Input: part model. Units: mm. Frame: model coordinates. A direction names the side the tool comes from. Round coordinates to 2 decimals unless told otherwise and drop trailing zeros. Loops run counter-clockwise (first coordinate to the right, second up) from the corner with the lowest first, then second, coordinate; pieces in that order, holes last. Notation, with made-up numbers: (59, -9.75) - (108, -9.75) arc R8 ccw to (108, -1.75) - close; hole circle Ø4 at (68, 2). An arc over 180 degrees is marked (long way). One line per question, with ' | ' between items. Start each with the question number.
Item 1: Section B-B, the plane z = 17.25. Return loops of the section in (x, y).
Item 2: Set-up query: faces 5 (the face through (17.5, -2, 14)), 6 (the face through (20.05, 11.9, 0.49)), 7 (the face through (0, -5, 23)), 8 (the face through (10, -3.4, 1)), 9 (the face through (0, -3, 3)). Return all of +Z, -Z, +X, -X, +Y, -Y with unobstructed straight access to the full face (end or side cutting, diameter ignored); none if empty.
Item 3: Section C-C, the plane z = 13. Return loops of the section in (x, y).
Item 4: Material intervals for line 1 along X through (y, z) = (1.25, 17.25); line 2 along X through (y, z) = (-3.5, 0.45); line 3 along Y through (x, z) = (12.5, 1.35), sorted ascending.
Item 5: Section D-D, the plane x = 31. Return loops of the section in (y, z), plus the area to 3 significant figures.
Item 6: Section A-A, the plane x = 8. Return loops of the section in (y, z).
Item 7: Draft query along Z for faces 1 (the face through (36.43, 7.4, 0.49)), 2 (the face through (19.68, -1.31, 2.87)), 3 (the face through (-16.5, -4, 10)), 4 (the face through (9, 0, 0)). Return one class per face: pulls with the +Z half, pulls with the -Z half, needs draft (parallel to the pull), parting line crosses it, or undercut.
Item 8: First-contact query: pin 1 (4 mm diameter, centred on x = 9, z = 17.5, fed in from +Y); pin 2 (0.8 mm diameter, centred on y = 2.5, z = 0.5, fed in from +X); pin 3 (6 mm diameter, centred on x = -4, z = 15.5, fed in from -Y). Flat tips, straight axial feed; report the tip coordinate or a pass-through.
```python
from build123d import *

# Parameters (mm, degrees)
INSERT_IN_SHEET_METAL_HOLE_DEPTH  = 1
BOSS_EXTRUDE5_DEPTH               = 1
SKETCH2_W                         = 24
SKETCH2_H                         = 2
LED_BACKING_DEPTH                 = 55
SKETCH3_R                         = 1
LED_SCREWHOLES_DEPTH              = 10
LED_BACKING_CLEANUP_DEPTH         = 52.613951602
LED_BACKING_CLEANUP_DEPTH_BACK    = 52.613951602
SKETCH5_W                         = 19.5
SKETCH5_H                         = 22
FILLET1_R                         = 3
BOSS_EXTRUDE3_START               = 5
BOSS_EXTRUDE3_DEPTH               = 5
FILLET2_R                         = 10
FILLET3_R                         = 5
FILLET4_R                         = 1
SKETCH7_R                         = 2.5
LED_WIRE_HOLES_DEPTH              = 51.714889332
SCREWHOLES_FOR_BACKING_DEPTH      = 51.714889332
SCREWHOLES_FOR_BACKING_DEPTH_BACK = 51.714889332
SKETCH8_R                         = 1
SKETCH9_W                         = 10
SKETCH9_H                         = 2
BOSS_EXTRUDE4_DEPTH               = 1
FILLET5_R                         = 3


with BuildPart() as part:
    # Sketch1 → Insert in sheet metal hole (new body)
    with BuildSketch(Plane.XY):
        with BuildLine():
            Line((-18, 11), (-18, -11))
            ThreePointArc((-18, -11), (-17.414213562, -12.414213562), (-16, -13))
            Line((-16, -13), (16, -13))
            ThreePointArc((16, -13), (20, -11.92820323), (22.92820323, -9))
            ThreePointArc((22.92820323, -9), (23.660254038, -8.267949192), (24.660254038, -8))
            Line((24.660254038, -8), (35, -8))
            ThreePointArc((35, -8), (36.414213562, -7.414213562), (37, -6))
            Line((37, -6), (37, 6))
            ThreePointArc((37, 6), (36.414213562, 7.414213562), (35, 8))
            Line((35, 8), (24.660254038, 8))
            ThreePointArc((24.660254038, 8), (23.660254038, 8.267949192), (22.92820323, 9))
            ThreePointArc((22.92820323, 9), (20, 11.92820323), (16, 13))
            Line((16, 13), (-16, 13))
            ThreePointArc((-16, 13), (-17.414213562, 12.414213562), (-18, 11))
        make_face()
    extrude(amount=INSERT_IN_SHEET_METAL_HOLE_DEPTH)

    # Sketch10 → Boss-Extrude5 (add)
    with BuildSketch(Plane.XY.offset(1)):
        with BuildLine():
            Line((26.246950766, -13), (35, -13))
            ThreePointArc((35, -13), (39.949747468, -10.949747468), (42, -6))
            Line((42, -6), (42, 6))
            ThreePointArc((42, 6), (39.949747468, 10.949747468), (35, 13))
            Line((35, 13), (26.246950766, 13))
            ThreePointArc((26.246950766, 13), (21.700877125, 16.683321446), (16, 18))
            Line((16, 18), (-16, 18))
            ThreePointArc((-16, 18), (-20.949747468, 15.949747468), (-23, 11))
            Line((-23, 11), (-23, -11))
            ThreePointArc((-23, -11), (-20.949747468, -15.949747468), (-16, -18))
            Line((-16, -18), (16, -18))
            ThreePointArc((16, -18), (21.700877125, -16.683321446), (26.246950766, -13))
        make_face()
    extrude(amount=BOSS_EXTRUDE5_DEPTH)

    # Sketch2 → LED backing (add)
    with BuildSketch(Plane.ZY.offset(18)):
        with Locations((12, 1)):
            Rectangle(SKETCH2_W, SKETCH2_H)
    extrude(amount=-LED_BACKING_DEPTH)

    # Sketch3 → LED screwholes (cut)
    with BuildSketch(Plane.XZ):
        with Locations(Location((-8, 17.25, 0), (0, 0, 270))):
            Circle(SKETCH3_R)
        with Locations(Location((8, 17.25, 0), (0, 0, 270))):
            Circle(SKETCH3_R)
    extrude(amount=-LED_SCREWHOLES_DEPTH, mode=Mode.SUBTRACT)

    # Sketch5 → LED backing cleanup (cut, two sides: drawn at the far end of the back side and taken through both)
    with BuildSketch(Plane.XZ.offset(-LED_BACKING_CLEANUP_DEPTH_BACK)):
        with Locations((27.25, 13)):
            Rectangle(SKETCH5_W, SKETCH5_H)
    extrude(amount=LED_BACKING_CLEANUP_DEPTH + LED_BACKING_CLEANUP_DEPTH_BACK, mode=Mode.SUBTRACT)

    # Fillet1
    fillet1_edges = [part.edges().sort_by_distance(p)[0] for p in [
        (17.5, 1, 24),
        (-18, 1, 24),
    ]]
    fillet(fillet1_edges, radius=FILLET1_R)

    # Sketch6 → Boss-Extrude3 (add)
    with BuildSketch(Plane.XZ.offset(BOSS_EXTRUDE3_START)):
        with BuildLine():
            Line((14.5, 24), (-15, 24))
            ThreePointArc((-15, 24), (-17.121320344, 23.121320344), (-18, 21))
            Line((-18, 21), (-18, 2))
            Line((-18, 2), (-16.5, 2))
            Line((-16.5, 2), (-16.5, 3.5))
            Line((-16.5, 3.5), (-16.5, 21))
            ThreePointArc((-16.5, 21), (-16.060660172, 22.060660172), (-15, 22.5))
            Line((-15, 22.5), (14.5, 22.5))
            ThreePointArc((14.5, 22.5), (15.560660172, 22.060660172), (16, 21))
            Line((16, 21), (16, 3.5))
            Line((16, 3.5), (16, 2))
            Line((16, 2), (17.5, 2))
            Line((17.5, 2), (17.5, 21))
            ThreePointArc((17.5, 21), (16.621320344, 23.121320344), (14.5, 24))
        make_face()
    extrude(amount=-BOSS_EXTRUDE3_DEPTH)

    # Fillet2
    fillet2_edges = [part.edges().sort_by_distance(p)[0] for p in [
        (-0.25, 2, 2),
        (-17.25, -5, 2),
        (16.75, -5, 2),
    ]]
    fillet(fillet2_edges, radius=FILLET2_R)

    # Fillet3
    fillet3_edges = [part.edges().sort_by_distance(p)[0] for p in [
        (17.5, -1.5, 2),
    ]]
    fillet(fillet3_edges, radius=FILLET3_R)

    # Fillet4
    fillet4_edges = [part.edges().sort_by_distance(p)[0] for p in [
        (-0.25, 0, 2),
        (-16.5, 0, 11.5),
        (-16.5, -7.5, 2),
        (-16.060660172, 0, 22.060660172),
        (-0.25, 0, 22.5),
        (15.560660172, 0, 22.060660172),
        (16, 0, 11.5),
        (16, -7.5, 2),
    ]]
    fillet(fillet4_edges, radius=FILLET4_R)

    # Sketch7 → LED wire holes (cut, through all)
    with BuildSketch(Plane.XY.offset(2)):
        with Locations((-13, -3.5)):
            Circle(SKETCH7_R)
        with Locations((12.5, -3.5)):
            Circle(SKETCH7_R)
    extrude(amount=-LED_WIRE_HOLES_DEPTH, mode=Mode.SUBTRACT)

    # Sketch8 → Screwholes for backing (cut, two sides: drawn at the far end of the back side and taken through both)
    with BuildSketch(Plane.XY.offset(2).offset(-SCREWHOLES_FOR_BACKING_DEPTH_BACK)):
        with Locations((0, -8)):
            Circle(SKETCH8_R)
        with Locations((-10, 8)):
            Circle(SKETCH8_R)
        with Locations((10, 8)):
            Circle(SKETCH8_R)
    extrude(amount=SCREWHOLES_FOR_BACKING_DEPTH + SCREWHOLES_FOR_BACKING_DEPTH_BACK, mode=Mode.SUBTRACT)

    # Sketch9 → Boss-Extrude4 (add)
    with BuildSketch(Plane.XY.offset(2)):
        with Locations((0, -2.75)):
            Rectangle(SKETCH9_W, SKETCH9_H)
    extrude(amount=BOSS_EXTRUDE4_DEPTH)

    # Fillet5
    # the kernel refuses this fillet: 3 mm, written as the material it adds along each edge
    with BuildSketch(Plane(origin=(5, -1.75, 2), x_dir=(1, 0, 0), z_dir=(0, -1, 0)), Plane(origin=(-5, -3.75, 2), x_dir=(-1, 0, 0), z_dir=(0, 1, 0))) as fillet5_piece_1:
        with BuildLine():
            CenterArc((2.236067977, 3), FILLET5_R, 221.810314896, 48.189685104)
            Line((0, 1), (0, 0))
            Line((0, 0), (2.236067977, 0))
        make_face()
    extrude(amount=2)
    with BuildSketch(Plane(origin=(5, -3.75, 2), x_dir=(0, -1, 0), z_dir=(-1, 0, 0))) as fillet5_piece_2:
        with BuildLine():
            CenterArc((2.236067977, 3), FILLET5_R, 221.810314896, 48.189685104)
            Line((0, 1), (0, 0))
            Line((0, 0), (2.236067977, 0))
        make_face()
    extrude(amount=10)
    with BuildSketch(Plane(origin=(10.590169944, -3.75, 2), x_dir=(0, -1, 0), z_dir=(-1, 0, 0))) as fillet5_piece_3a_section:
        with BuildLine():
            CenterArc((2.236067977, 3), FILLET5_R, 221.810314896, 48.189685104)
            Line((0, 1), (0, 0))
            Line((0, 0), (2.236067977, 0))
        make_face()
    fillet5_piece_3a = extrude(amount=15.590169944, mode=Mode.PRIVATE)
    fillet5_piece_3a = fillet5_piece_3a - Plane(origin=(12.5, -3.5, 2), x_dir=(1, 0, 0), z_dir=(0, 0, 1)) * Cylinder(2.5, 41, mode=Mode.PRIVATE)
    fillet5_piece_3a = split(fillet5_piece_3a, bisect_by=Plane(origin=(5, -3.75, 2), z_dir=(1, 0, 0)), keep=Keep.TOP, mode=Mode.PRIVATE)
    with BuildSketch(Plane(origin=(5, -1.75, 2), x_dir=(1, 0, 0), z_dir=(0, -1, 0))) as fillet5_piece_3b_section:
        with BuildLine():
            CenterArc((2.236067977, 3), FILLET5_R, 221.810314896, 48.189685104)
            Line((0, 1), (0, 0))
            Line((0, 0), (2.236067977, 0))
        make_face()
    fillet5_piece_3b = extrude(amount=7.590169944, mode=Mode.PRIVATE)
    fillet5_piece_3b = split(fillet5_piece_3b, bisect_by=Plane(origin=(5, -3.75, 2), z_dir=(0, -1, 0)), keep=Keep.TOP, mode=Mode.PRIVATE)
    fillet5_piece_3 = fillet5_piece_3a & fillet5_piece_3b
    add(fillet5_piece_3)
    with BuildSketch(Plane(origin=(-5, -9.340169944, 2), x_dir=(-1, 0, 0), z_dir=(0, 1, 0))) as fillet5_piece_4a_section:
        with BuildLine():
            CenterArc((2.236067977, 3), FILLET5_R, 221.810314896, 48.189685104)
            Line((0, 1), (0, 0))
            Line((0, 0), (2.236067977, 0))
        make_face()
    fillet5_piece_4a = extrude(amount=7.590169944, mode=Mode.PRIVATE)
    fillet5_piece_4a = split(fillet5_piece_4a, bisect_by=Plane(origin=(-5, -3.75, 2), z_dir=(0, -1, 0)), keep=Keep.TOP, mode=Mode.PRIVATE)
    with BuildSketch(Plane(origin=(5, -3.75, 2), x_dir=(0, -1, 0), z_dir=(-1, 0, 0))) as fillet5_piece_4b_section:
        with BuildLine():
            CenterArc((2.236067977, 3), FILLET5_R, 221.810314896, 48.189685104)
            Line((0, 1), (0, 0))
            Line((0, 0), (2.236067977, 0))
        make_face()
    fillet5_piece_4b = extrude(amount=15.590169944, mode=Mode.PRIVATE)
    fillet5_piece_4b = split(fillet5_piece_4b, bisect_by=Plane(origin=(-5, -3.75, 2), z_dir=(-1, 0, 0)), keep=Keep.TOP, mode=Mode.PRIVATE)
    fillet5_piece_4b = fillet5_piece_4b - Plane(origin=(-13, -3.5, 2), x_dir=(1, 0, 0), z_dir=(0, 0, 1)) * Cylinder(2.5, 41, mode=Mode.PRIVATE)
    fillet5_piece_4 = fillet5_piece_4a & fillet5_piece_4b
    add(fillet5_piece_4)


solid = part.part
```
Return value:
1) outline: (-18, -5) - (-16.5, -5) - (-16.5, -1) arc R1 cw to (-15.5, 0) - (-9, 0) - (-9, 2) - (-18, 2) - close; (-7, 0) - (7, 0) - (7, 2) - (-7, 2) - close; (9, 0) - (15, 0) arc R1 cw to (16, -1) - (16, -5) - (17.5, -5) - (17.5, 2) - (9, 2) - close
2) face 5: +Z, +X, +Y, -Y | face 6: -Z, +X, +Y | face 7: +Z, +X, -X, -Y | face 8: -Z | face 9: -Y
3) outline: (-18, -5) - (-16.5, -5) - (-16.5, -1) arc R1 cw to (-15.5, 0) - (15, 0) arc R1 cw to (16, -1) - (16, -5) - (17.5, -5) - (17.5, 2) - (-18, 2) - close
4) line 1: -18 to -9, -7 to 7, 9 to 17.5 | line 2: -18 to -15.5, -10.5 to 10, 15 to 37 | line 3: -18 to -6, -1 to 18
5) outline: (-13, 1) - (-8, 1) - (-8, 0) - (8, 0) - (8, 1) - (13, 1) - (13, 2) - (-13, 2) - close | area: 42.0 mm2
6) outline: (-18, 1) - (-13, 1) - (-13, 0) - (13, 0) - (13, 1) - (18, 1) - (18, 2) - (12, 2) arc R10 cw to (2, 12) - (2, 16.25) - (0, 16.25) - (0, 3) arc R1 cw to (-1, 2) - (-18, 2) - close; (-5, 22.5) - (-1, 22.5) arc R1 cw to (0, 21.5) - (0, 18.25) - (2, 18.25) - (2, 24) - (-5, 24) - close
7) face 1: needs draft | face 2: pulls with the +Z half | face 3: undercut | face 4: pulls with the -Z half
8) pin 1: y = 2 | pin 2: x = 37 | pin 3: y = 0
